Geometry check sheet. Reference: drawing and pictorial views, mm from the part's lowest x, y, z. Coordinates: 2 decimals unless noted, no trailing zeros. Loops run counter-clockwise (first coordinate to the right, second up) from the corner with the lowest first, then second, coordinate; pieces in that order, holes last. Notation, with made-up numbers: (72.5, -31.75) - (124.5, -31.75) arc R27 ccw to (124.5, -6.75) - close; hole circle Ø8 at (48, 66). An arc over 180 degrees is marked (long way). One line per item, written item: value.
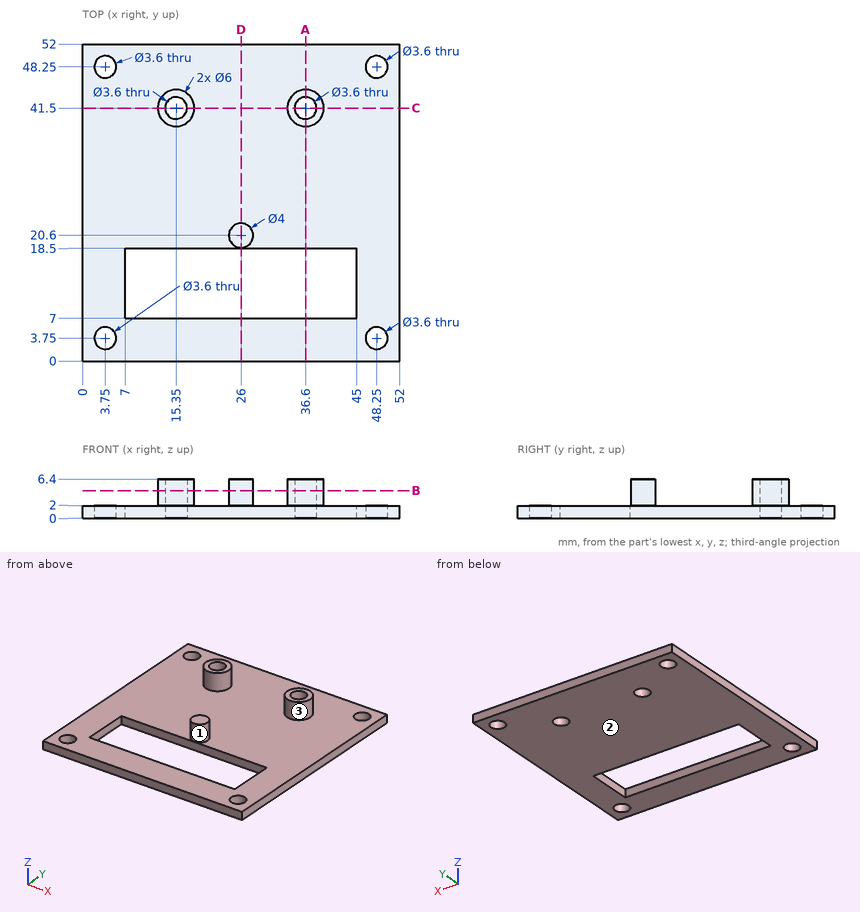
(1) Material ranges on probe 1 along Y at (x, z) = (48.25, 1.05); probe 2 along Y at (x, z) = (11.5, 1); probe 3 along Z at (x, y) = (10, 50), recorded low to high. Write a range as from..to.
Reply:
probe 1: 0..1.95, 5.55..46.45, 50.05..52
probe 2: 0..7, 18.5..52
probe 3: 0..2
(2) Go/stop test with flat-tipped pins: pin 1 Ø4 at (x, y) = (3.75, 48.25) entering from +Z; pin 2 Ø3 at (x, y) = (48.25, 48.25) entering from +Z. Record where each tip stops, or that it passes through.
Reply:
pin 1: z = 2
pin 2: through
(3) Release check for a two-part mould opening along X. For the marked faces 1, 2 and 3 record: pulls with the +X half, pulls with the -X half, needs draft (parallel to the pull), parting line crosses it, or undercut.
Reply:
face 1: parting line crosses it
face 2: needs draft
face 3: undercut
(4) Cross-section at B-B on z = 4.5. Record the cut outline in (x, y), and give its area (3 significant figures).
Reply:
outline: circle Ø6 at (15.35, 41.5); circle Ø4 at (26, 20.6); circle Ø6 at (36.6, 41.5); hole circle Ø3.6 at (15.35, 41.5); hole circle Ø3.6 at (36.6, 41.5)
area: 48.8 mm2
(5) Cross-section at D-D on x = 26. Record the cut outline in (y, z).
Reply:
outline: (0, 0) - (7, 0) - (7, 2) - (0, 2) - close; (18.5, 0) - (52, 0) - (52, 2) - (22.6, 2) - (22.6, 6.4) - (18.6, 6.4) - (18.6, 2) - (18.5, 2) - close
(6) Cross-section at C-C on y = 41.5. Record the cut outline in (x, z), and give its area (3 significant figures).
Reply:
outline: (0, 0) - (13.55, 0) - (13.55, 6.4) - (12.35, 6.4) - (12.35, 2) - (0, 2) - close; (17.15, 0) - (34.8, 0) - (34.8, 6.4) - (33.6, 6.4) - (33.6, 2) - (18.35, 2) - (18.35, 6.4) - (17.15, 6.4) - close; (38.4, 0) - (52, 0) - (52, 2) - (39.6, 2) - (39.6, 6.4) - (38.4, 6.4) - close
area: 111 mm2
(7) Cross-section at A-A on x = 36.6. Record the cut outline in (y, z), and give its area (3 significant figures).
Reply:
outline: (0, 0) - (7, 0) - (7, 2) - (0, 2) - close; (18.5, 0) - (39.7, 0) - (39.7, 6.4) - (38.5, 6.4) - (38.5, 2) - (18.5, 2) - close; (43.3, 0) - (52, 0) - (52, 2) - (44.5, 2) - (44.5, 6.4) - (43.3, 6.4) - close
area: 84.4 mm2
